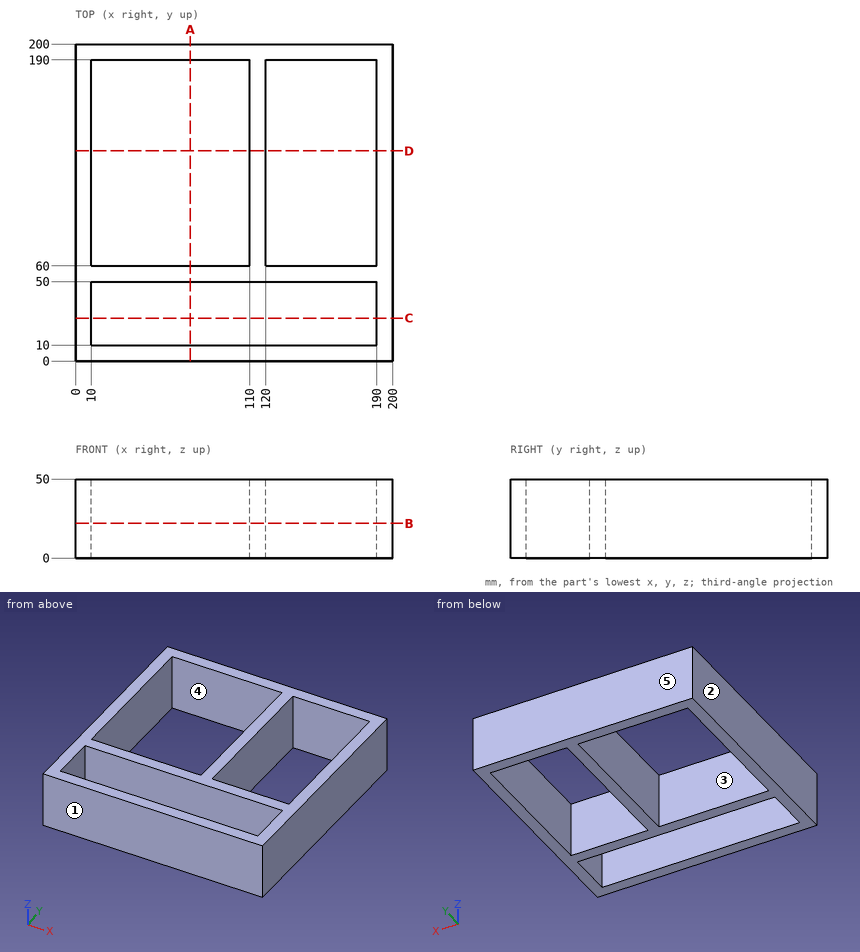
The drawing under review shows one solid part. Ordinate dimensions are in mm from its lowest x, y, z. A direction names the side the tool comes from. Round coordinates to 2 decimals unless told otherwise and drop trailing zeros. Write each loop counter-clockwise with the first axis right and the second up, starting at its lowest first coordinate (ties: lowest second). Pieces come first, ordered by that corner, then holes. Notation, with made-up numbers: M 55.25,35.25 L 94.25,35.25 A17 ccw 94.25,66.25 Z; hole C 36,37 d2. An arc over 180 degrees is marked long. One line per item, written item: value. Start each with the question number.
(1) We need section A-A (x = 72.5). Give the boundary of the cut face in (y, z), and give its area (3 significant figures).
(2) Wall thickness on line 1 (Y direction, x = 121, z = 8); line 2 (X direction, y = 156, z = 5); line 3 (X direction, y = 32.5, z = 31.5): over which ranges is each line inside the solid? List them lowest first.
(3) We need section C-C (y = 27). Give the boundary of the cut face in (x, z).
(4) The part is to be moulded in two halves that separate along Y. For the marked faces 1, 2 and 3, say which applies: released by +Y, released by -Y, zero draft, split by the parting line, or undercut.
(5) Machinability: for the marked faces 4 and 5, which of the approach directions +Z, -Z, +X, -X, +Y, -Y give a long, thin tool a straight path to every point of the face, cutting with its end or side? Answer none if there is none.
(6) We need section B-B (z = 22). Give the boundary of the cut face in (x, y).
(7) We need section D-D (y = 132.5). Give the boundary of the cut face in (x, z), and give its area (3 significant figures).
Result:
1. outline: M 0,0 L 10,0 L 10,50 L 0,50 Z; M 50,0 L 60,0 L 60,50 L 50,50 Z; M 190,0 L 200,0 L 200,50 L 190,50 Z
1. area: 1,500 mm²
2. line 1: 0 to 10, 50 to 60, 190 to 200
2. line 2: 0 to 10, 110 to 120, 190 to 200
2. line 3: 0 to 10, 190 to 200
3. outline: M 0,0 L 10,0 L 10,50 L 0,50 Z; M 190,0 L 200,0 L 200,50 L 190,50 Z
4. face 1: released by -Y
4. face 2: zero draft
4. face 3: undercut
5. face 4: +Z, -Z
5. face 5: +Z, -Z, +X, -X, +Y
6. outline: M 0,0 L 200,0 L 200,200 L 0,200 Z; hole M 10,10 L 190,10 L 190,50 L 10,50 Z; hole M 10,60 L 110,60 L 110,190 L 10,190 Z; hole M 120,60 L 190,60 L 190,190 L 120,190 Z
7. outline: M 0,0 L 10,0 L 10,50 L 0,50 Z; M 110,0 L 120,0 L 120,50 L 110,50 Z; M 190,0 L 200,0 L 200,50 L 190,50 Z
7. area: 1,500 mm²
